Design review of the part built by this model. Coordinates are the model's own, in mm. Face numbers are marked on the shaded views. A direction names the side the tool comes from. Give positions to 0.01 mm unless a question says otherwise; leave off trailing zeros. Loops run counter-clockwise (first coordinate to the right, second up) from the corner with the lowest first, then second, coordinate; pieces in that order, holes last. Notation, with made-up numbers: M 16,-25 L 66,-25 A20 cw 66,5 Z; hole C -9,1 d11. An arc over 180 degrees is marked long. Use CSV: the item, a comma, the result in double quotes.
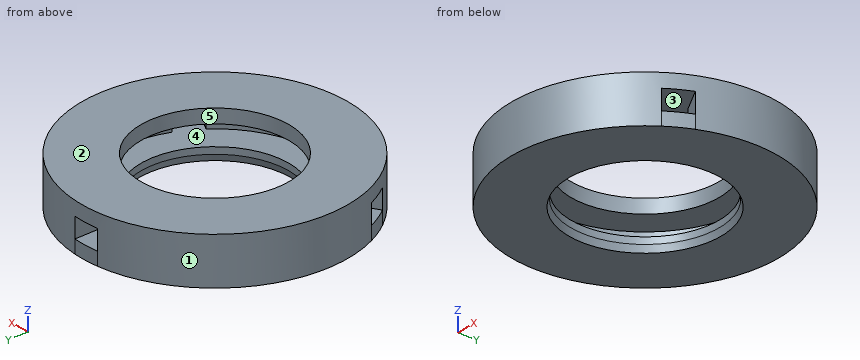
from build123d import *

# Parameters (mm, degrees)
F0_R     = 20
F0_R_2   = 11.1125
F1_DEPTH = 7.1
F2_R     = 11.1125
F3_DEPTH = 5
F4_R     = 11.1125
F5_DEPTH = 2
F6_SIZE2 = 1
F6_SIZE  = 0.3


with BuildPart() as f1:
    # F0 (on Top) → F1 (new body)
    with BuildSketch(Plane.XY):
        Circle(F0_R)
        Circle(F0_R_2, mode=Mode.SUBTRACT)
    extrude(amount=F1_DEPTH)

    # F2 (on Top) → F3 (cut)
    with BuildSketch(Plane.XY):
        with BuildLine():
            Line((-2, 19.899749), (-2, 15.370426))
            ThreePointArc((-2, 15.370426), (-13.423394, 7.75), (-14.31118, -5.953162))
            Line((-14.31118, -5.953162), (-18.233688, -8.217824))
            ThreePointArc((-18.233688, -8.217824), (-17.320508, -10), (-16.233688, -11.681925))
            Line((-16.233688, -11.681925), (-12.31118, -9.417264))
            ThreePointArc((-12.31118, -9.417264), (0, -15.5), (12.31118, -9.417264))
            Line((12.31118, -9.417264), (16.233688, -11.681925))
            ThreePointArc((16.233688, -11.681925), (17.320508, -10), (18.233688, -8.217824))
            Line((18.233688, -8.217824), (14.31118, -5.953162))
            ThreePointArc((14.31118, -5.953162), (13.423394, 7.75), (2, 15.370426))
            Line((2, 15.370426), (2, 19.899749))
            ThreePointArc((2, 19.899749), (0, 20), (-2, 19.899749))
        make_face()
        Circle(F2_R, mode=Mode.SUBTRACT)
    extrude(amount=F3_DEPTH, mode=Mode.SUBTRACT)

    # F4 (on Top) → F5 (join)
    with BuildSketch(Plane.XY):
        with BuildLine():
            Line((-2, 19.899749), (-2, 15.370426))
            ThreePointArc((-2, 15.370426), (-13.423394, 7.75), (-14.31118, -5.953162))
            Line((-14.31118, -5.953162), (-18.233688, -8.217824))
            ThreePointArc((-18.233688, -8.217824), (-17.320508, -10), (-16.233688, -11.681925))
            Line((-16.233688, -11.681925), (-12.31118, -9.417264))
            ThreePointArc((-12.31118, -9.417264), (0, -15.5), (12.31118, -9.417264))
            Line((12.31118, -9.417264), (16.233688, -11.681925))
            ThreePointArc((16.233688, -11.681925), (17.320508, -10), (18.233688, -8.217824))
            Line((18.233688, -8.217824), (14.31118, -5.953162))
            ThreePointArc((14.31118, -5.953162), (13.423394, 7.75), (2, 15.370426))
            Line((2, 15.370426), (2, 19.899749))
            ThreePointArc((2, 19.899749), (0, 20), (-2, 19.899749))
        make_face()
        Circle(F4_R, mode=Mode.SUBTRACT)
    extrude(amount=F5_DEPTH)

    # F6
    f6_edges = [f1.edges().sort_by_distance(p)[0] for p in [
        (-11.1125, 0, 0),
    ]]
    chamfer(f6_edges, length=F6_SIZE, length2=F6_SIZE2)


solid = f1.part
(1) We need section C-C on z = 4.25. State the section outline as (x, y) points.
A:
outline,"M -18.23,-8.22 L -14.31,-5.95 A15.5 cw -2,15.37 L -2,19.9 A20 ccw Z; M -16.23,-11.68 A20 ccw 16.23,-11.68 L 12.31,-9.42 A15.5 cw -12.31,-9.42 Z; M 2,15.37 A15.5 cw 14.31,-5.95 L 18.23,-8.22 A20 ccw 2,19.9 Z"
(2) We need section D-D on z = 0.5. State the section outline as (x, y) points (1 decimal), then the cut area to 3 significant figures.
A:
outline,"M -18.2,-8.2 A20 ccw -16.2,-11.7 A20 ccw 16.2,-11.7 A20 ccw 18.2,-8.2 A20 ccw 2,19.9 A20 ccw -2,19.9 A20 ccw Z; hole C 0,0 d22.5"
area,"858 mm²"
(3) Clearance check with flat-ended pins moving along their axes: P1, Ø18, axis at x = 0, y = 0, coming from the +Z side; P2, Ø1.5, axis at x = 0, z = 2.5, coming from the +Y side; P3, Ø2, axis at y = 16, z = 1.5, coming from the -X side; P4, Ø4, axis at x = -6.5, z = 4, coming from the +Y side. State where each tip first meets the part, or that it passes through.
A:
P1,"through"
P2,"y = 20"
P3,"x = -13.23"
P4,"y = 19.49"
(4) We need section B-B on x = 0. State the section outline as (y, z) points, then the cut area to 3 significant figures.
A:
outline,"M -20,0 L -11.41,0 L -11.11,1 L -11.11,2 L -15.5,2 L -15.5,5 L -11.11,5 L -11.11,7.1 L -20,7.1 Z; M 11.11,1 L 11.41,0 L 20,0 L 20,2 L 11.11,2 Z; M 11.11,5 L 20,5 L 20,7.1 L 11.11,7.1 Z"
area,"86.1 mm²"
(5) We need section A-A on y = 0. State the section outline as (x, z) points.
A:
outline,"M -20,0 L -11.41,0 L -11.11,1 L -11.11,2 L -15.5,2 L -15.5,5 L -11.11,5 L -11.11,7.1 L -20,7.1 Z; M 11.11,1 L 11.41,0 L 20,0 L 20,7.1 L 11.11,7.1 L 11.11,5 L 15.5,5 L 15.5,2 L 11.11,2 Z"
(6) Machinability: for the marked faces 4 and 5, which of the approach directions +Z, -Z, +X, -X, +Y, -Y give a long, thin tool a straight path to every point of the face, cutting with its end or side? Answer none if there is none.
A:
face 4,"none"
face 5,"+Z, -Z"
(7) Wall thickness on line 1 along Z through (x, y) = (6, 11); line 2 along Y through (x, z) = (0, 1.3); line 3 along X through (y, z) = (1, 1.75): over which ranges is each line inside the solid? List them lowest first. Write a range as [from, to].
A:
line 1,"[0, 2], [5, 7.1]"
line 2,"[-20, -11.11], [11.11, 20]"
line 3,"[-19.97, -11.07], [11.07, 19.97]"
(8) The part is to be moulded in two halves that separate along Y. For the marked faces 1, 2 and 3, say which applies: released by +Y, released by -Y, zero draft, split by the parting line, or undercut.
A:
face 1,"split by the parting line"
face 2,"zero draft"
face 3,"undercut"
